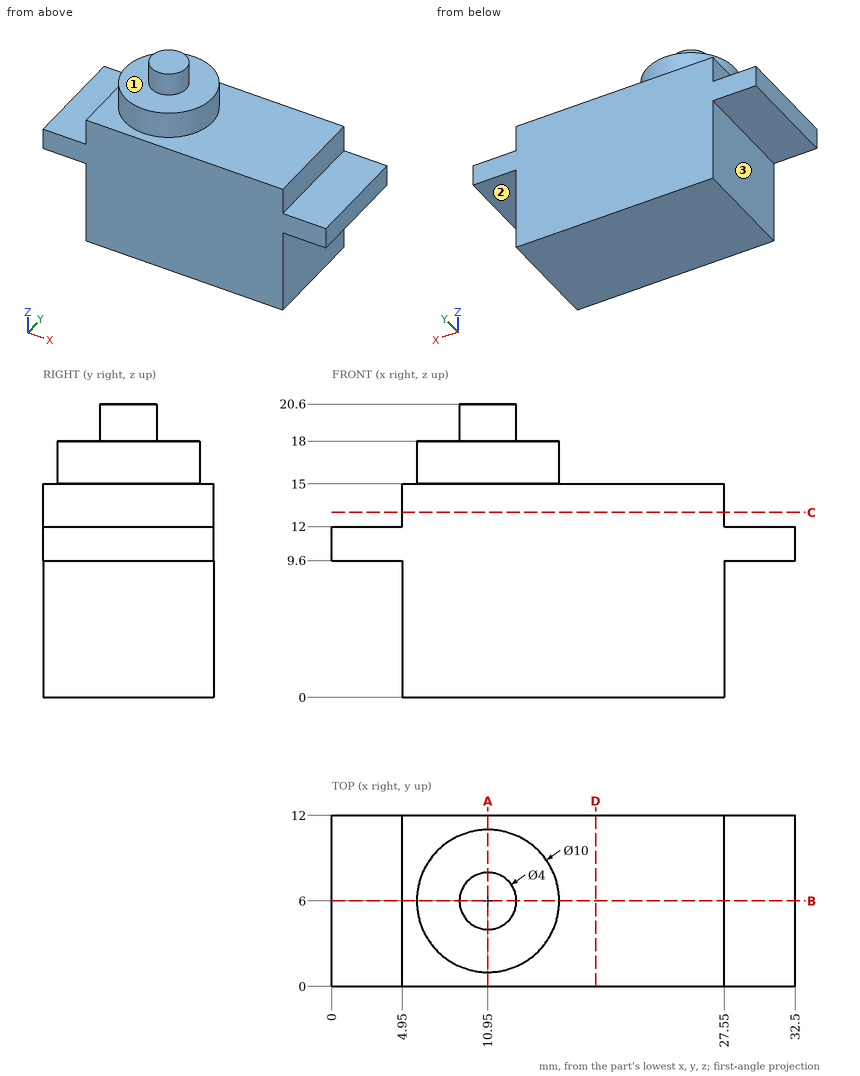
The figure shows three views and two pictorial views of one solid part (mm, origin at its lowest corner). Answer the questions. A direction names the side the tool comes from. Coordinates: 2 decimals unless noted, no trailing zeros. Loops run counter-clockwise (first coordinate to the right, second up) from the corner with the lowest first, then second, coordinate; pieces in that order, holes last. Notation, with made-up numbers: (44.25, 34.25) -> (68.25, 34.25) arc R32 ccw to (68.25, 65.25) -> close; hole circle Ø2 at (66, 84). An arc over 180 degrees is marked (long way). Use one line per item in the form item = value. Start each with the question number.
Item 1: Consider L1, parallel to X at y = 5.75, z = 16.75; L2, parallel to Z at x = 11.5, y = 11.25; L3, parallel to X at y = 6.5, z = 1.5. Determine where each line is inside the solid, lowest interval first. Write a range as [from, to].
Item 2: A tool of negligible diameter and unlimited length cuts with its end or side. For the marked faces 1, 2 and 3, from which of +Z, -Z, +X, -X, +Y, -Y can it reach the whole face along a straight path? Write none if from no direction.
Item 3: The part is cut by section C-C on z = 13. Determine the outline of the cut face in (x, y), then the cut area to 3 significant figures.
Item 4: The part is cut by section A-A on x = 10.95. Determine the outline of the cut face in (y, z), then the cut area to 3 significant figures.
Item 5: The part is cut by section B-B on y = 6. Determine the outline of the cut face in (x, z), then the cut area to 3 significant figures.
Item 6: The part is cut by section D-D on x = 18.5. Determine the outline of the cut face in (y, z).
Item 7: Flat-ended cylindrical pins translate along their axes: pin 1 Ø4 at (y, z) = (9, 15.5) entering from +X; pin 2 Ø5 at (x, y) = (24, 1.5) entering from -Z; pin 3 Ø5 at (y, z) = (5.5, 5) entering from -X; pin 4 Ø5.5 at (x, y) = (31, 4.5) entering from +Z. Find the tip coordinate at first contact, or state that the pin passes through.
Answer key:
q1.L1 = [5.96, 15.94]
q1.L2 = [0, 15]
q1.L3 = [4.95, 27.55]
q2.face_1 = +Z
q2.face_2 = -Z, +X, +Y, -Y
q2.face_3 = -Z, -X, +Y, -Y
q3.outline = (4.95, 0) -> (27.55, 0) -> (27.55, 12) -> (4.95, 12) -> close
q3.area = 271 mm2
q4.outline = (0, 0) -> (12, 0) -> (12, 15) -> (11, 15) -> (11, 18) -> (8, 18) -> (8, 20.6) -> (4, 20.6) -> (4, 18) -> (1, 18) -> (1, 15) -> (0, 15) -> close
q4.area = 220 mm2
q5.outline = (0, 9.6) -> (4.95, 9.6) -> (4.95, 0) -> (27.55, 0) -> (27.55, 9.6) -> (32.5, 9.6) -> (32.5, 12) -> (27.55, 12) -> (27.55, 15) -> (15.95, 15) -> (15.95, 18) -> (12.95, 18) -> (12.95, 20.6) -> (8.95, 20.6) -> (8.95, 18) -> (5.95, 18) -> (5.95, 15) -> (4.95, 15) -> (4.95, 12) -> (0, 12) -> close
q5.area = 403 mm2
q6.outline = (0, 0) -> (12, 0) -> (12, 15) -> (0, 15) -> close
q7.pin_1 = 27.55
q7.pin_2 = 0
q7.pin_3 = 4.95
q7.pin_4 = 12
